Design review of the part shown in the three views and the two pictorial views. Dimensions are in mm from the part's minimum x, y and z. A direction names the side the tool comes from. Round coordinates to 2 decimals unless told otherwise and drop trailing zeros. Loops run counter-clockwise (first coordinate to the right, second up) from the corner with the lowest first, then second, coordinate; pieces in that order, holes last. Notation, with made-up numbers: M -29.75,66 L 6.25,66 A27 cw 6.25,86 Z; hole C -3.5,61 d2. An arc over 180 degrees is marked long. Return JSON: item names as keys, results as strings. Group by question number.
Q1. Consider section A-A (z = 11). State the section outline as (x, y) points.
Q2. Consider section C-C (y = 80.5). State the section outline as (x, z) points.
Q3. Consider section B-B (x = 55). State the section outline as (y, z) points, and give its area (3 significant figures).
Q4. Clearance check with flat-ended pins moving along their axes: pin 1 Ø6.5 at (y, z) = (43.5, 13) entering from -X; pin 2 Ø11 at (y, z) = (48, 13.5) entering from +X; pin 3 Ø11 at (x, z) = (91, 13) entering from +Y. State where each tip first meets the part, or that it passes through.
Q5. Consider section D-D (x = 80). State the section outline as (y, z) points.
Q6. For the marked faces 1, 2 and 3, list the 3-axis set-ups (+Z, -Z, +X, -X, +Y, -Y) from which the entire face can be reached by the end or side of a thin tool; tool diameter is ignored.
Q7. To check wall thickness, follow line 1 along Y through (x, z) = (54.5, 18); line 2 along Y through (x, z) = (23, 1.5); line 3 along X through (y, z) = (61.5, 14.75). State the ranges of each line that lie inside material, in increasing order.
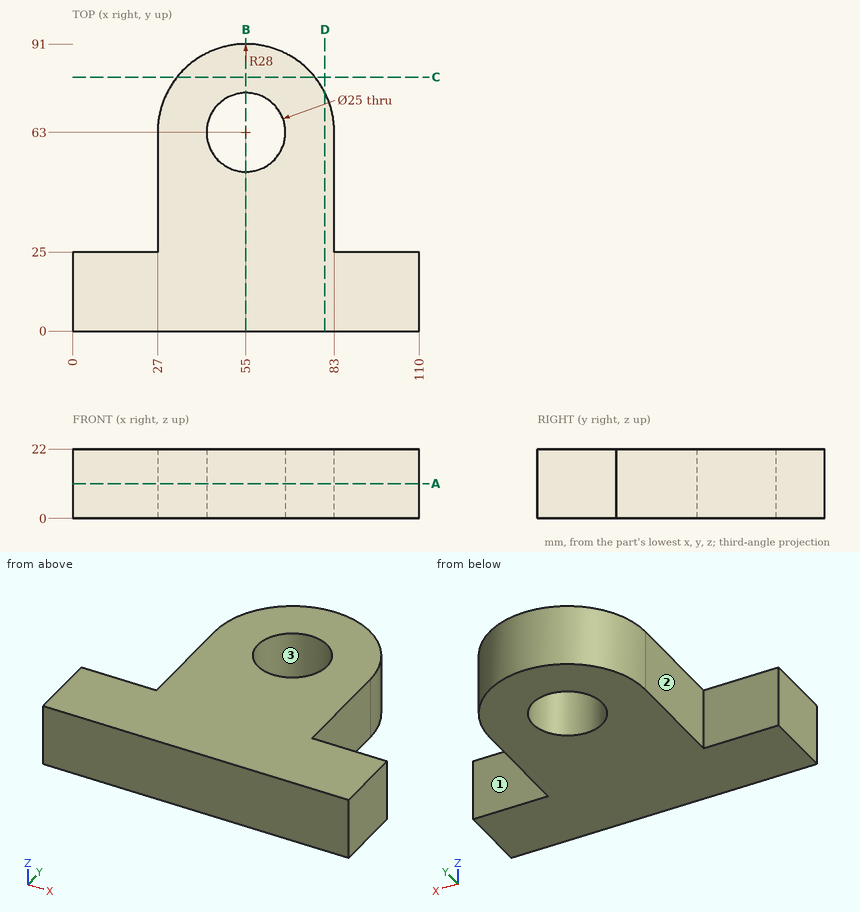
Values:
{
 "1": {"outline": "M 0,0 L 110,0 L 110,25 L 83,25 L 83,63 A28 ccw 27,63 L 27,25 L 0,25 Z; hole C 55,63 d25"},
 "2": {"outline": "M 33.14,0 L 76.86,0 L 76.86,22 L 33.14,22 Z"},
 "3": {"outline": "M 0,0 L 50.5,0 L 50.5,22 L 0,22 Z; M 75.5,0 L 91,0 L 91,22 L 75.5,22 Z", "area": "1,450 mm2"},
 "4": {"pin 1": "stops at x = 27", "pin 2": "stops at x = 83", "pin 3": "stops at y = 25"},
 "5": {"outline": "M 0,0 L 75.61,0 L 75.61,22 L 0,22 Z"},
 "6": {"face 1": "+Z, -Z, +X, +Y", "face 2": "+Z, -Z, -X, +Y", "face 3": "+Z, -Z"},
 "7": {"line 1": "y = 0 to 50.51, 75.49 to 91", "line 2": "y = 0 to 25", "line 3": "x = 27 to 42.59, 67.41 to 83"}
}
